Check sheet for the modelled part. Datum: model origin and axes. Units: mm. Coordinates: 2 decimals unless noted, no trailing zeros. Loops run counter-clockwise (first coordinate to the right, second up) from the corner with the lowest first, then second, coordinate; pieces in that order, holes last. Notation, with made-up numbers: M 20,45.5 L 39,45.5 A25 cw 39,61.5 Z; hole C -1.5,-26.75 d4. An arc over 180 degrees is marked long. Use CSV: the item, a comma, the result in double quotes. Start each with the question number.
(1) Section check A-A on x = -6.5. Record the cut outline in (y, z), and give its area (3 significant figures).
(2) Section check D-D on z = 0. Record the cut outline in (x, y), and give its area (3 significant figures).
(3) Section check C-C on z = 15. Record the cut outline in (x, y), and give its area (3 significant figures).
(4) Scan lines: line 1 (X direction, y = 1.15, z = 0); line 2 (X direction, y = 2.7, z = 15); line 3 (X direction, y = 0.2, z = -17). Record each from-to range of solid material in increasing order.
(5) Section check B-B on y = 2.1. Record the cut outline in (x, z).
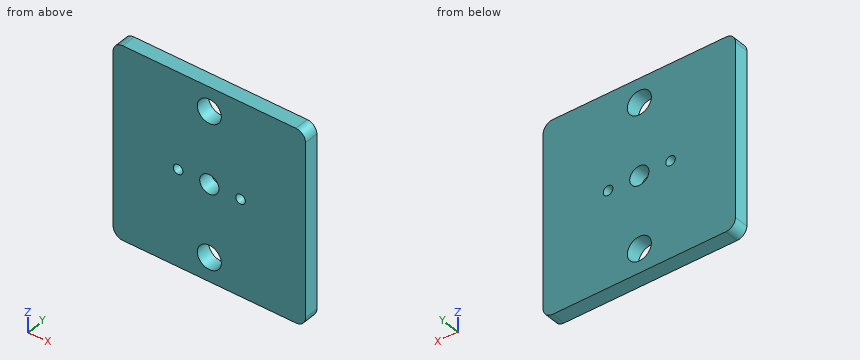
from build123d import *

# Parameters (mm, degrees)
BOSS_EXTRUDE1_DEPTH = 3
SKETCH3_R           = 2
SKETCH3_R_2         = 2.5
CUT_EXTRUDE3_DEPTH  = 29.442925307
SKETCH4_R           = 1
CUT_EXTRUDE4_DEPTH  = 3


with BuildPart() as part:
    # Sketch2 → Boss-Extrude1 (new body)
    with BuildSketch(Plane(origin=(0, 0, 0), x_dir=(1, 0, 0), z_dir=(0, 1, 0))):
        with BuildLine():
            Line((-18, -20), (18, -20))
            ThreePointArc((18, -20), (19.414213562, -19.414213562), (20, -18))
            Line((20, -18), (20, 18))
            ThreePointArc((20, 18), (19.414213562, 19.414213562), (18, 20))
            Line((18, 20), (-18, 20))
            ThreePointArc((-18, 20), (-19.414213562, 19.414213562), (-20, 18))
            Line((-20, 18), (-20, -18))
            ThreePointArc((-20, -18), (-19.414213562, -19.414213562), (-18, -20))
        make_face()
    extrude(amount=BOSS_EXTRUDE1_DEPTH)

    # Sketch3 → Cut-Extrude3 (cut, through all)
    with BuildSketch(Plane(origin=(0, 0, 0), x_dir=(1, 0, 0), z_dir=(0, 1, 0))):
        with Locations(Location((0, 0, 0), (0, 0, 270))):
            Circle(SKETCH3_R)
        with Locations(Location((0, 15, 0), (0, 0, 270))):
            Circle(SKETCH3_R_2)
        with Locations(Location((0, -15, 0), (0, 0, 270))):
            Circle(SKETCH3_R_2)
    extrude(amount=CUT_EXTRUDE3_DEPTH, mode=Mode.SUBTRACT)

    # Sketch4 → Cut-Extrude4 (cut)
    with BuildSketch(Plane(origin=(0, 0, 0), x_dir=(1, 0, 0), z_dir=(0, 1, 0))):
        with Locations(Location((6.5, 0, 0), (0, 0, 270))):
            Circle(SKETCH4_R)
        with Locations(Location((-6.5, 0, 0), (0, 0, 270))):
            Circle(SKETCH4_R)
    extrude(amount=CUT_EXTRUDE4_DEPTH, mode=Mode.SUBTRACT)


solid = part.part
Outcome:
1,outline,"M 0,-20 L 3,-20 L 3,-1 L 0,-1 Z; M 0,1 L 3,1 L 3,20 L 0,20 Z"
1,area,"114 mm²"
2,outline,"M -20,0 L -7.5,0 L -7.5,3 L -20,3 Z; M -5.5,0 L -2,0 L -2,3 L -5.5,3 Z; M 2,0 L 5.5,0 L 5.5,3 L 2,3 Z; M 7.5,0 L 20,0 L 20,3 L 7.5,3 Z"
2,area,"96.0 mm²"
3,outline,"M -20,0 L -2.5,0 L -2.5,3 L -20,3 Z; M 2.5,0 L 20,0 L 20,3 L 2.5,3 Z"
3,area,"105 mm²"
4,line 1,"x = -20 to -7.5, -5.5 to -2, 2 to 5.5, 7.5 to 20"
4,line 2,"x = -20 to -2.5, 2.5 to 20"
4,line 3,"x = -20 to -1.5, 1.5 to 20"
5,outline,"M -20,-18 A2 ccw -18,-20 L 18,-20 A2 ccw 20,-18 L 20,18 A2 ccw 18,20 L -18,20 A2 ccw -20,18 Z; hole C -6.5,0 d2; hole C 0,-15 d5; hole C 0,15 d5; hole C 0,0 d4; hole C 6.5,0 d2"
